from build123d import *

# Parameters (mm, degrees)
BOSS_EXTRUDE1_DEPTH = 152.4
CHAMFER1_SIZE       = 0.254


with BuildPart() as part:
    # Sketch1 → Boss-Extrude1 (new body)
    with BuildSketch(Plane(origin=(0, 0, 0), x_dir=(-1, 0, 0), z_dir=(0, 0, -1))):
        Polygon((3.666174209, 6.35), (-3.666174209, 6.35), (-7.332348419, 0), (-3.666174209, -6.35), (3.666174209, -6.35), (7.332348419, 0), align=None)
    extrude(amount=-BOSS_EXTRUDE1_DEPTH)

    # Chamfer1
    chamfer1_edges = [part.edges().sort_by_distance(p)[0] for p in [
        (5.499261314, 3.175, 152.4),
        (5.499261314, -3.175, 152.4),
        (0, -6.35, 152.4),
        (-5.499261314, -3.175, 152.4),
        (-5.499261314, 3.175, 152.4),
        (-5.499261314, -3.175, 0),
        (0, -6.35, 0),
        (5.499261314, -3.175, 0),
        (5.499261314, 3.175, 0),
        (0, 6.35, 0),
        (-5.499261314, 3.175, 0),
        (0, 6.35, 152.4),
    ]]
    chamfer(chamfer1_edges, length=CHAMFER1_SIZE)


solid = part.part
Model file for the job. Use its own axes, mm. Give positions to 0.01 mm unless a question says otherwise; leave off trailing zeros. Write each loop counter-clockwise with the first axis right and the second up, starting at its lowest first coordinate (ties: lowest second). Pieces come first, ordered by that corner, then holes. Notation, with made-up numbers: (31.25, 70.5) -> (60.25, 70.5) arc R16 ccw to (60.25, 87.5) -> close; hole circle Ø8 at (-6.5, 85.5). An arc over 180 degrees is marked (long way). Write item = value, one per line.
(1) Probe line 1 along X through (y, z) = (1, 83.5) (3 decimals); line 2 along X through (y, z) = (5.5, 86.5); line 3 along Y through (x, z) = (6, 39.5). List the from-to ranges inside material, lowest first.
Determined:
line_1 = -6.755 to 6.755
line_2 = -4.16 to 4.16
line_3 = -2.31 to 2.31
(2) Slice it at C-C, the plane y = -2.75. Give the cut face in (x, z).
Determined:
outline = (-5.74, 0.25) -> (-5.45, 0) -> (5.45, 0) -> (5.74, 0.25) -> (5.74, 152.15) -> (5.45, 152.4) -> (-5.45, 152.4) -> (-5.74, 152.15) -> close
(3) Flat gauge pins, fed straight in: P1, Ø1.5, axis at y = -3.5, z = 115.5, coming from the +X side; P2, Ø1, axis at x = -4.5, z = 31, coming from the +Y side; P3, Ø2, axis at y = 3, z = 124.5, coming from the -X side. Where does each tip first touch, or does it go through?
Determined:
P1 = 5.74
P2 = 5.77
P3 = -6.18
(4) Slice it at B-B, the plane x = 5.5. Give the cut face in (y, z), then the cut area to 3 significant figures.
Determined:
outline = (-3.17, 0.25) -> (-2.67, 0) -> (2.67, 0) -> (3.17, 0.25) -> (3.17, 152.15) -> (2.67, 152.4) -> (-2.67, 152.4) -> (-3.17, 152.15) -> close
area = 967 mm2
(5) Slice it at A-A, the plane z = 94.5. Give the cut face in (x, y).
Determined:
outline = (-7.33, 0) -> (-3.67, -6.35) -> (3.67, -6.35) -> (7.33, 0) -> (3.67, 6.35) -> (-3.67, 6.35) -> close
